```python
from build123d import *

# Parameters (mm, degrees)
F0_R      = 39.9
F1_DEPTH  = 4
F2_R      = 29
F3_DEPTH  = 4
F4_R      = 31
F5_DEPTH  = 30
F5_FACE_R = 29
F6_DEPTH  = 26
F8_R      = 2
F9_DEPTH  = 4
F11_R     = 2
F12_DEPTH = 4
F13_R     = 2.5
F14_DEPTH = 4
F16_DEPTH = 2.4


with BuildPart() as f1:
    # F0 (on Top) → F1 (new body)
    with BuildSketch(Plane.XY):
        Circle(F0_R)
    extrude(amount=F1_DEPTH)

    # F2 (on face) → F3 (cut)
    with BuildSketch(Plane.XY.offset(4)):
        Circle(F2_R)
    extrude(amount=-F3_DEPTH, mode=Mode.SUBTRACT)

    # F4 (on face) → F5 (join)
    with BuildSketch(Plane.XY.offset(4)):
        Circle(F4_R)
    extrude(amount=F5_DEPTH)

    # F5_face (on face) → F6 (cut)
    with BuildSketch(Plane(origin=(0, 0, 4), x_dir=(1, 0, 0), z_dir=(0, 0, -1))):
        Circle(F5_FACE_R)
    extrude(amount=-F6_DEPTH, mode=Mode.SUBTRACT)

    # F8 (on face) → F9 (cut)
    with BuildSketch(Plane(origin=(0, 0, 0), x_dir=(1, 0, 0), z_dir=(0, 0, -1))):
        with Locations((-23.645058, -24.431767)):
            Circle(F8_R)
        with Locations((-9.336002, 32.693104)):
            Circle(F8_R)
        with Locations((32.98106, -8.261338)):
            Circle(F8_R)
    extrude(amount=-F9_DEPTH, mode=Mode.SUBTRACT)

    # F11 (on face) → F12 (cut)
    with BuildSketch(Plane.XY.offset(34)):
        with Locations((18, 18)):
            Circle(F11_R)
        with Locations((-18, 18)):
            Circle(F11_R)
        with Locations((-18, -18)):
            Circle(F11_R)
        with Locations((18, -18)):
            Circle(F11_R)
    extrude(amount=-F12_DEPTH, mode=Mode.SUBTRACT)

    # F13 (on face) → F14 (cut)
    with BuildSketch(Plane.XY.offset(34)):
        with Locations((0, -1)):
            Circle(F13_R)
    extrude(amount=-F14_DEPTH, mode=Mode.SUBTRACT)

    # F15 (on face) → F16 (cut)
    with BuildSketch(Plane.XY.offset(34)):
        Polygon((15.45842, -19.903603), (18.377779, -21.152874), (20.919359, -19.249271), (20.54158, -16.096397), (17.622221, -14.847126), (15.080641, -16.750729), align=None)
        Polygon((-20.61525, -19.801056), (-17.747865, -21.165401), (-15.132615, -19.364345), (-15.38475, -16.198944), (-18.252135, -14.834599), (-20.867385, -16.635655), align=None)
        Polygon((14.975065, 16.994466), (17.35189, 14.888751), (20.363905, 15.894285), (20.999095, 19.005534), (18.622269, 21.111249), (15.610254, 20.105715), align=None)
        Polygon((-20.066176, 15.588725), (-16.944863, 15.005001), (-14.878686, 17.416276), (-15.933824, 20.411275), (-19.055137, 20.994999), (-21.121314, 18.583724), align=None)
    extrude(amount=-F16_DEPTH, mode=Mode.SUBTRACT)


solid = f1.part
```
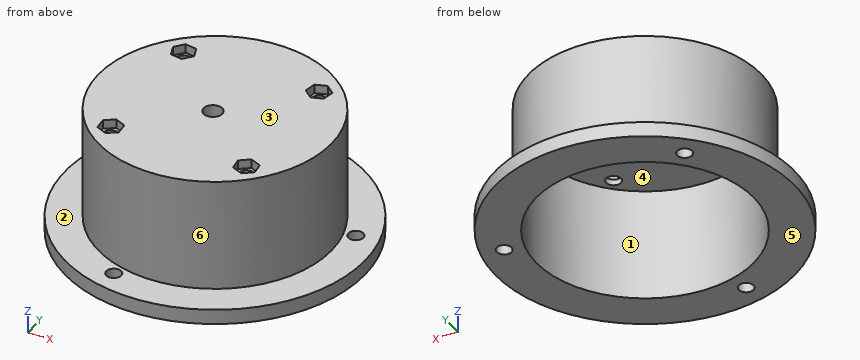
For this review, take the finished solid that the model builds, in its own axes (mm). Face numbers are marked on the shaded views. A direction names the side the tool comes from. Give positions to 0.01 mm unless a question says otherwise; leave off trailing zeros. Order: outer loops, then holes, each group sorted by start corner. A loop starts at its lowest first (then second) coordinate and runs counter-clockwise, first axis right, second up.
1) The part is to be moulded in two halves that separate along X. For the marked faces 4, 5 and 6, say which applies: released by +X, released by -X, zero draft, split by the parting line, or undercut.
2) Take a section at B-B (y = -18). Give the boundary of the cut face in (x, z), then the cut area to 3 significant figures.
3) Take a section at C-C (z = 11.5). Give the boundary of the cut face in (x, y).
4) Take a section at A-A (x = 0). Give the boundary of the cut face in (y, z).
5) Take a section at D-D (y = -1). Give the boundary of the cut face in (x, z), then the cut area to 3 significant figures.
6) Insertion check: pin 1 (4.5 mm diameter, centred on x = 18, y = 18, fed in from +Z); pin 2 (12 mm diameter, centred on x = 14, y = -13.5, fed in from -Z); pin 3 (2.5 mm diameter, centred on x = -9.34, y = -32.69, fed in from +Z); pin 4 (1 mm diameter, centred on x = 1, z = 9, fed in from +Y). Each pin has a flat end and moves straight along its axis. Give the tip position at first contact, or say it passes through.
7) Wall thickness on line 1 (X direction, y = 25, z = 2); line 2 (X direction, y = -17, z = 20); line 3 (X direction, y = -18, z = 32): over which ranges is each line inside the solid? List them lowest first.
8) For the marked faces 1, 2 and 3, list the 3-axis set-ups (+Z, -Z, +X, -X, +Y, -Y) from which the entire face can be reached by the end or side of a thin tool; tool diameter is ignored.
Derived:
1. face 4: undercut
1. face 5: zero draft
1. face 6: split by the parting line
2. outline: (-35.61, 0) - (-22.74, 0) - (-22.74, 30) - (-20, 30) - (-20, 31.6) - (-20.76, 31.6) - (-20.76, 34) - (-25.24, 34) - (-25.24, 4) - (-35.61, 4) - close; (-16, 30) - (16, 30) - (16, 31.6) - (15.23, 31.6) - (15.23, 34) - (-15.24, 34) - (-15.24, 31.6) - (-16, 31.6) - close; (20, 30) - (22.74, 30) - (22.74, 0) - (35.61, 0) - (35.61, 4) - (25.24, 4) - (25.24, 34) - (20.77, 34) - (20.77, 31.6) - (20, 31.6) - close
2. area: 396 mm2
3. outline: circle Ø62 at (0, 0); hole circle Ø58 at (0, 0)
4. outline: (-39.9, 0) - (-29, 0) - (-29, 30) - (-3.5, 30) - (-3.5, 34) - (-31, 34) - (-31, 4) - (-39.9, 4) - close; (1.5, 30) - (29, 30) - (29, 0) - (39.9, 0) - (39.9, 4) - (31, 4) - (31, 34) - (1.5, 34) - close
5. outline: (-39.89, 0) - (-28.98, 0) - (-28.98, 30) - (-2.5, 30) - (-2.5, 34) - (-30.98, 34) - (-30.98, 4) - (-39.89, 4) - close; (2.5, 30) - (28.98, 30) - (28.98, 0) - (39.89, 0) - (39.89, 4) - (30.98, 4) - (30.98, 34) - (2.5, 34) - close
5. area: 419 mm2
6. pin 1: stops at z = 31.6
6. pin 2: stops at z = 30
6. pin 3: passes through
6. pin 4: stops at y = 31
7. line 1: x = -31.1 to -25.56, -21.73 to -14.7, 14.7 to 31.1
7. line 2: x = -25.92 to -23.49, 23.49 to 25.92
7. line 3: x = -25.24 to -20.76, -15.24 to 15.23, 20.77 to 25.24
8. face 1: -Z
8. face 2: +Z
8. face 3: +Z, +X, -X, +Y, -Y
